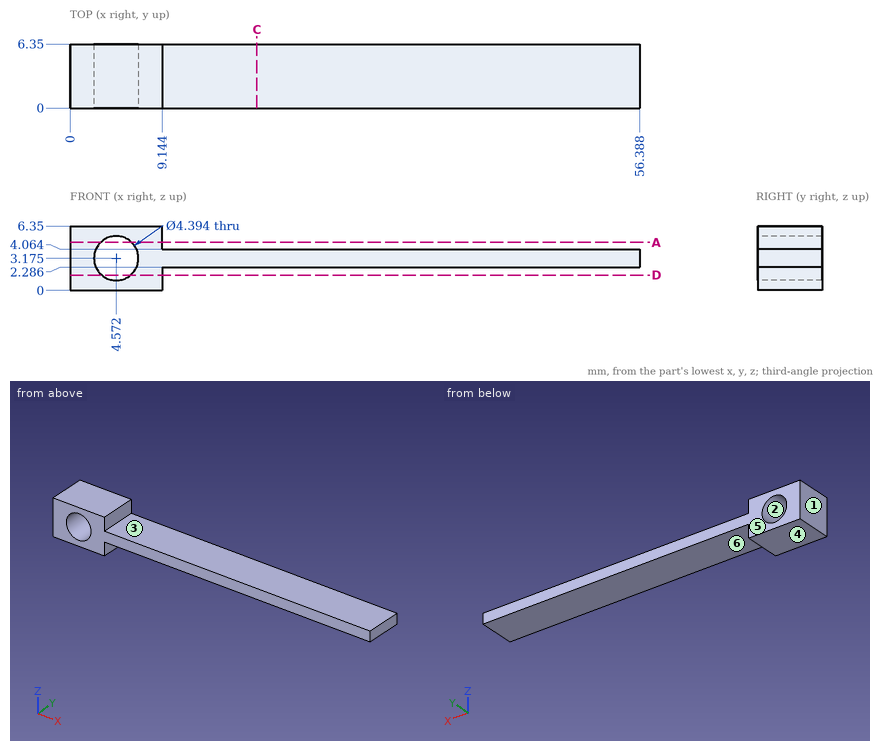
Here's the drawing with two shaded views (mm, measured from the low corner). I have some questions. A direction names the side the tool comes from. Coordinates: 2 decimals unless noted, no trailing zeros. Order: outer loops, then holes, each group sorted by start corner. A loop starts at its lowest first (then second) coordinate and runs counter-clockwise, first axis right, second up. Notation, with made-up numbers: (27, 64) - (86, 64) arc R7 ccw to (86, 68) - close; hole circle Ø10 at (2.5, 61). An arc over 180 degrees is marked (long way). Answer in a Markdown table with one row per item.
1. If I drill on line 1 along Z through (x, y) = (50, 3.25); line 2 along X through (y, z) = (0.75, 4.75) (1 decimal); line 3 along X through (y, z) = (4, 4.5) (1 decimal), over which ranges is the centre line in solid material (lowest first)?
Reply:
| item | result |
|---|---|
| line 1 | z = 2.29 to 4.06 |
| line 2 | x = 0 to 3, 6.1 to 9.1 |
| line 3 | x = 0 to 2.8, 6.3 to 9.1 |
2. Suppose I cut it at D-D (z = 1.5). Please give me the cut outline in (x, y).
Reply:
| item | result |
|---|---|
| outline | (0, 0) - (3.15, 0) - (3.15, 6.35) - (0, 6.35) - close; (5.99, 0) - (9.14, 0) - (9.14, 6.35) - (5.99, 6.35) - close |
3. For pin 1 (1.5 mm diameter, centred on x = 36.5, y = 3.5, fed in from +Z); pin 2 (1.8 mm diameter, centred on y = 4, z = 5, fed in from +X), each with a flat end and sliding along its axis, tell me the tip position at first contact or that it passes through.
Reply:
| item | result |
|---|---|
| pin 1 | stops at z = 4.06 |
| pin 2 | stops at x = 9.14 |
4. Suppose I cut it at C-C (x = 18.5). Please give me the cut outline in (y, z), and give its area (3 significant figures).
Reply:
| item | result |
|---|---|
| outline | (0, 2.29) - (6.35, 2.29) - (6.35, 4.06) - (0, 4.06) - close |
| area | 11.3 mm^2 |
5. For the marked faces 5 and 6, which set-ups out of +Z, -Z, +X, -X, +Y, -Y let a thin tool reach every point of the face, with its end or its side?
Reply:
| item | result |
|---|---|
| face 5 | +Z, -Z, +X, -X, +Y |
| face 6 | -Z, +X, +Y, -Y |
6. Suppose I cut it at A-A (z = 4.75). Please give me the cut outline in (x, y), and give its area (3 significant figures).
Reply:
| item | result |
|---|---|
| outline | (0, 0) - (3.04, 0) - (3.04, 6.35) - (0, 6.35) - close; (6.1, 0) - (9.14, 0) - (9.14, 6.35) - (6.1, 6.35) - close |
| area | 38.6 mm^2 |
7. If we mould it in two halves opening along Z, with no side actions, what happens to the marked faces 1, 2, 3 and 4? For each: pulls with the +Z half, pulls with the -Z half, needs draft (parallel to the pull), parting line crosses it, or undercut.
Reply:
| item | result |
|---|---|
| face 1 | needs draft |
| face 2 | undercut |
| face 3 | pulls with the +Z half |
| face 4 | pulls with the -Z half |
